CAD build for the part. Positions are in the model's coordinates, mm. A direction names the side the tool comes from. Round coordinates to 2 decimals unless told otherwise and drop trailing zeros. Order: outer loops, then holes, each group sorted by start corner. A loop starts at its lowest first (then second) coordinate and runs counter-clockwise, first axis right, second up.
```python
from build123d import *

# Parameters (mm, degrees)
BOSS_EXTRUDE1_DEPTH = 2.5
SKETCH6_R           = 2
CUT_EXTRUDE2_DEPTH  = 81.683428275
FILLET1_R           = 10
FILLET2_R           = 0.25
CUT_EXTRUDE3_DEPTH  = 1
CUT_EXTRUDE3_DRAFT  = -45
FILLET3_R           = 10


# Read off the part's stored shape, not the designer's step: Mirror1
with BuildPart() as part:
    # Sketch5 → Boss-Extrude1 (new, symmetric)
    with BuildSketch(Plane(origin=(0, 0, 0), x_dir=(1, 0, 0), z_dir=(0, 1, 0))):
        with BuildLine():
            Line((-32.965704319, 40.746204167), (-5.742345952, 60.760614197))
            ThreePointArc((-5.742345952, 60.760614197), (2.206223968, 68.07965732), (3, 57.303847577))
            Line((3, 57.303847577), (3, 5.196152423))
            ThreePointArc((3, 5.196152423), (2.317397773, -5.534407607), (-5.807325554, 1.508300339))
            Line((-5.807325554, 1.508300339), (-34.741264584, 30.00061646))
            ThreePointArc((-34.741264584, 30.00061646), (-42.258431929, 36.762212041), (-32.965704319, 40.746204167))
        make_face()
    extrude(amount=BOSS_EXTRUDE1_DEPTH, both=True)

    # Sketch6 → Cut-Extrude2 (cut, through all)
    with BuildSketch(Plane(origin=(0, 2.5, 0), x_dir=(1, 0, 0), z_dir=(0, 1, 0))):
        with Locations(Location((-36.338700951, 35.784058087, 0), (0, 0, 270))):
            Circle(SKETCH6_R)
        with Locations(Location((0, 62.5, 0), (0, 0, 270))):
            Circle(SKETCH6_R)
        with Locations(Location((0, 0, 0), (0, 0, 270))):
            Circle(SKETCH6_R)
    extrude(amount=-CUT_EXTRUDE2_DEPTH, mode=Mode.SUBTRACT)

    # Fillet1
    fillet1_edges = [part.edges().sort_by_distance(p)[0] for p in [
        (3, 0, -57.303847577),
        (3, 0, -5.196152423),
        (-5.807325554, 0, -1.508300339),
        (-34.741264584, 0, -30.00061646),
        (-32.965704319, 0, -40.746204167),
        (-5.742345952, 0, -60.760614197),
    ]]
    fillet(fillet1_edges, radius=FILLET1_R)

    # Fillet2
    fillet2_edges = [part.edges().sort_by_distance(p)[0] for p in [
        (2.317397773, -2.5, 5.534407607),
        (2.317397773, 2.5, 5.534407607),
        (-20.274295069, -2.5, -15.754458399),
        (-20.274295069, 2.5, -15.754458399),
        (-42.294061571, -2.5, -36.514592059),
        (-42.294061571, 2.5, -36.514592059),
        (-19.354025135, -2.5, -50.753409182),
        (-19.354025135, 2.5, -50.753409182),
        (2.436899667, -2.5, -67.982838682),
        (2.436899667, 2.5, -67.982838682),
        (3, -2.5, -31.25),
        (3, 2.5, -31.25),
        (-6.906263042, -2.5, -1.916404592),
        (-6.906263042, 2.5, -1.916404592),
        (-34.316307366, -2.5, -28.908085432),
        (-34.316307366, 2.5, -28.908085432),
        (-32.227862875, -2.5, -42.090278775),
        (-32.227862875, 2.5, -42.090278775),
        (-7.245317265, -2.5, -60.457259979),
        (-7.245317265, 2.5, -60.457259979),
        (3.480283618, -2.5, -56.234483125),
        (3.480283618, 2.5, -56.234483125),
        (3.480283618, -2.5, -6.265516875),
        (3.480283618, 2.5, -6.265516875),
    ]]
    fillet(fillet2_edges, radius=FILLET2_R)


with BuildPart() as cut_extrude3_tool:
    # Sketch11 → Cut-Extrude3 (with draft: the straight prism first)
    with BuildSketch(Plane(origin=(0, 2.5, 0), x_dir=(1, 0, 0), z_dir=(0, 1, 0))):
        with BuildLine():
            ThreePointArc((-30.596355, 37.52344389), (-30.339901547, 35.904081877), (-30.531375397, 34.275757748))
            Line((-30.531375397, 34.275757748), (-3, 7.164597728))
            Line((-3, 7.164597728), (-3, 57.812078262))
            Line((-3, 57.812078262), (-30.596355, 37.52344389))
        make_face()
    extrude(amount=-CUT_EXTRUDE3_DEPTH)
    # Cut-Extrude3: the draft: its side faces are tilted about the plane it starts from
    cut_extrude3_sides = [cut_extrude3_tool.faces().sort_by_distance(p)[0] for p in [
        (-30.339901547, 2, -35.904081877),
        (-16.765687699, 2, -20.720177738),
        (-3, 2, -32.488337995),
        (-16.7981775, 2, -47.667761076),
    ]]
    draft(cut_extrude3_sides, Plane(origin=(0, 2.5, 0), x_dir=(1, 0, 0), z_dir=(0, 1, 0)), CUT_EXTRUDE3_DRAFT)


with BuildPart() as part_1:
    add(part.part)

    # Cut-Extrude3: cut by cut_extrude3_tool
    add(cut_extrude3_tool.part, mode=Mode.SUBTRACT)

    # Fillet3
    # the kernel refuses this fillet: 10 mm, written as the material it adds along each edge
    with BuildSketch(Plane(origin=(-35.422208483, 1.5, -40.495403727), x_dir=(-0.4961401986594238, 0.7071067811865456, 0.5038302325924777), z_dir=(0.712523548065871, 0, 0.701648197782637))) as fillet3_piece_1_section:
        with BuildLine():
            CenterArc((4.695967592, -9.446168032), FILLET3_R, 109.158067237, 25.841932763)
            Line((-2.37510022, -2.37510022), (0, 0))
            Line((0, 0), (1.414213562, 0))
        make_face()
    fillet3_piece_1 = extrude(amount=52.497135101, mode=Mode.PRIVATE)
    fillet3_piece_1 = split(fillet3_piece_1, bisect_by=Plane(origin=(-21.679167278, -8.239532903, -30.749685658), z_dir=(0.4188457426606433, 0.7071067811865488, 0.5697089115110034)), keep=Keep.TOP, mode=Mode.PRIVATE)
    fillet3_piece_1 = split(fillet3_piece_1, bisect_by=Plane(origin=(-9.768964958, -4.268964958, -22.714341228), z_dir=(-0.7071067811865462, 0.7071067811865488, 0)), keep=Keep.TOP, mode=Mode.PRIVATE)
    add(fillet3_piece_1)
    with BuildSketch(Plane(origin=(2.765578806, 1.5, -60.809716743), x_dir=(-0.4188457426606457, 0.7071067811865447, -0.5697089115110068), z_dir=(-0.805690069263676, 0, 0.5923373298129141))) as fillet3_piece_2_section:
        with BuildLine():
            CenterArc((4.695967592, -9.446168032), FILLET3_R, 109.158067237, 25.841932763)
            Line((-2.37510022, -2.37510022), (0, 0))
            Line((0, 0), (1.414213562, 0))
        make_face()
    fillet3_piece_2 = extrude(amount=48.40225373, mode=Mode.PRIVATE)
    fillet3_piece_2 = split(fillet3_piece_2, bisect_by=Plane(origin=(-9.835247725, -4.335247725, -45.695753356), z_dir=(-0.7071067811865462, 0.7071067811865488, 0)), keep=Keep.TOP, mode=Mode.PRIVATE)
    add(fillet3_piece_2)
    with BuildSketch(Plane(origin=(-4, 1.5, -1.155549611), x_dir=(0.7071067811865488, 0.7071067811865462, 0), z_dir=(0, 0, -1))) as fillet3_piece_3_section:
        with BuildLine():
            CenterArc((4.695967592, -9.446168032), FILLET3_R, 109.158067237, 25.841932763)
            Line((-2.37510022, -2.37510022), (0, 0))
            Line((0, 0), (1.414213562, 0))
        make_face()
    fillet3_piece_3 = extrude(amount=63.077411412, mode=Mode.PRIVATE)
    fillet3_piece_3 = split(fillet3_piece_3, bisect_by=Plane(origin=(-10.603901171, -7.527129797, -39.776353526), z_dir=(0.4188457426606433, 0.7071067811865488, 0.5697089115110034)), keep=Keep.TOP, mode=Mode.PRIVATE)
    fillet3_piece_3 = split(fillet3_piece_3, bisect_by=Plane(origin=(-10.614934948, -6.100094299, -26.733213697), z_dir=(0.49614019865942166, 0.7071067811865488, -0.5038302325924754)), keep=Keep.TOP, mode=Mode.PRIVATE)
    add(fillet3_piece_3)

    # Mirror1
    split(bisect_by=Plane.ZX, keep=Keep.TOP)

    # Mirror1 2: part across plane


with BuildPart() as part_2:
    add(part_1.part)
    add(part_1.part.mirror(Plane.ZX))


solid = part_2.part
```
1. Mould opens along X. For faces 1 (the face through (3, 0, -32)), 2 (the face through (-2, -2.5, -31)), 3 (the face through (-15.7, 1.76, -22.6)) say: released by +X, released by -X, zero draft, split by the parting line, or undercut.
2. Cut at A-A, the plane y = 0.7. Write the cut outline in (x, z) (3 decimals).
3. Cut at B-B, the plane x = 0. Give the number of separate pieces and of enclosed holes in the cut face, and give its area (3 significant figures).
4. Pin check, flat tips, straight feed: P1, Ø6.5, axis at x = 0, z = -62.5, coming from the -Y side; P2, Ø1, axis at x = -7.5, z = -29.5, coming from the -Y side; P3, Ø1.3, axis at y = 0.5, z = -33, coming from the +X side; P4, Ø9, axis at x = -18, z = -39, coming from the +Y side. Stop position of each tip, or through.
5. Drill centre lines: line 1 (Z direction, x = 4, y = 2.25); line 2 (X direction, y = 0.8, z = 0); line 3 (X direction, y = 1.2, z = -62.5). Where is each one in solid material? Low to high.
6. Tool access for faces 4 (the face through (-5.09, 1.76, -32.13)), 5 (the face through (-5.09, -1.76, -32.13)), 6 (the face through (3.467, 0.031, -6.307)): list every direction of +Z, -Z, +X, -X, +Y, -Y with a clear straight run to the whole face (end or side of a thin tool).
Outcome:
1. face 1: released by +X
1. face 2: zero draft
1. face 3: undercut
2. outline: (-37.267, -29.856) arc R6 ccw to (-35.807, -41.76) arc R10 cw to (-28.997, -43.664) - (-9.711, -57.843) arc R10 cw to (-5.863, -63.775) arc R6 ccw (long way) to (4.875, -59.002) arc R10 cw to (3, -53.173) - (3, -9.327) arc R10 cw to (4.875, -3.498) arc R6 ccw (long way) to (-5.913, 1.019) arc R10 cw to (-8.751, -4.407) - (-31.798, -27.102) arc R10 cw to start; hole circle Ø4 at (-36.339, -35.784); hole circle Ø4 at (0, -62.5); hole circle Ø4 at (0, 0)
3. separate pieces: 3
3. enclosed holes: 0
3. area: 332 mm2
4. P1: stops at y = -2.5
4. P2: stops at y = -1.51
4. P3: stops at x = 3
4. P4: stops at y = 1.84
5. line 1: z = -66.97 to -57.53, -4.97 to 4.47
5. line 2: x = -6.14 to -2, 2 to 6
5. line 3: x = -6.23 to -2, 2 to 6
6. face 4: +Y
6. face 5: -Y
6. face 6: +X, +Y, -Y
